Geometry check sheet. Reference: the model listing, model coordinates, mm. Face numbers are marked on the shaded views. A direction names the side the tool comes from. Give positions to 0.01 mm unless a question says otherwise; leave off trailing zeros. Order: outer loops, then holes, each group sorted by start corner. A loop starts at its lowest first (then second) coordinate and runs counter-clockwise, first axis right, second up. Notation, with made-up numbers: M 47.25,-26.5 L 61.25,-26.5 A21 cw 61.25,-13.5 Z; hole C 43,55.5 d10. An arc over 180 degrees is marked long. Answer as CSV lines item,"result".
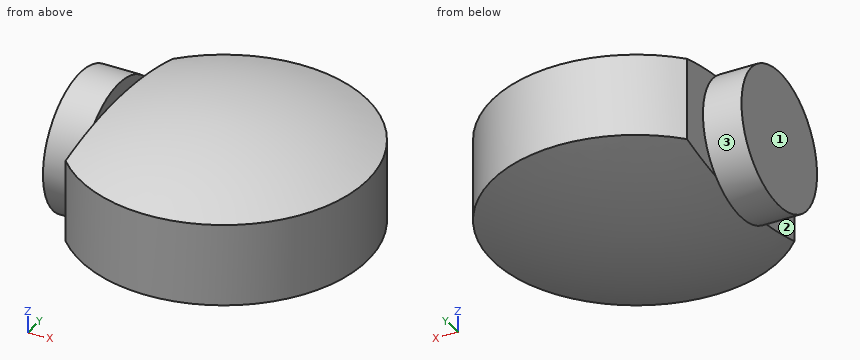
from build123d import *

# Parameters (mm, degrees)
ESQUISSE1_R           = 26
EXTRUSION1_DEPTH      = 15
D_ME1_FACE_RADIUS     = 26
D_ME1_HEIGHT          = 5
D_ME2_FACE_RADIUS     = 26
D_ME2_HEIGHT          = 5
EXTRUSION2_DEPTH      = 42.856899073
EXTRUSION2_DEPTH_BACK = 42.856899073
ESQUISSE2_W           = 16.897481419
ESQUISSE2_H           = 62.481047215
ESQUISSE3_R           = 12.5
EXTRUSION3_DEPTH      = 7


with BuildPart() as part:
    # Esquisse1 → Extrusion1 (new body)
    with BuildSketch(Plane.XY):
        Circle(ESQUISSE1_R)
    extrude(amount=EXTRUSION1_DEPTH)

    # Dôme1: a dome of height H over a round flat face of radius A is a cap of a sphere of radius (A * A + H * H) / (2 * H)
    d_me1_r = (D_ME1_FACE_RADIUS * D_ME1_FACE_RADIUS + D_ME1_HEIGHT * D_ME1_HEIGHT) / (2 * D_ME1_HEIGHT)
    d_me1_base = Plane((0, 0, 15), z_dir=(0, 0, 1))
    with Locations(d_me1_base.offset(D_ME1_HEIGHT - d_me1_r)):
        d_me1_ball = Sphere(d_me1_r, mode=Mode.PRIVATE)
    add(split(d_me1_ball, bisect_by=d_me1_base, keep=Keep.TOP, mode=Mode.PRIVATE))

    # Dôme2: a dome of height H over a round flat face of radius A is a cap of a sphere of radius (A * A + H * H) / (2 * H)
    d_me2_r = (D_ME2_FACE_RADIUS * D_ME2_FACE_RADIUS + D_ME2_HEIGHT * D_ME2_HEIGHT) / (2 * D_ME2_HEIGHT)
    d_me2_base = Plane((0, 0, 0), z_dir=(0, 0, -1))
    with Locations(d_me2_base.offset(D_ME2_HEIGHT - d_me2_r)):
        d_me2_ball = Sphere(d_me2_r, mode=Mode.PRIVATE)
    add(split(d_me2_ball, bisect_by=d_me2_base, keep=Keep.TOP, mode=Mode.PRIVATE))

    # Esquisse2 → Extrusion2 (cut, two sides: drawn at the far end of the back side and taken through both)
    with BuildSketch(Plane.XY.offset(-EXTRUSION2_DEPTH_BACK)):
        with Locations((-27.44874071, 0.855485378)):
            Rectangle(ESQUISSE2_W, ESQUISSE2_H)
    extrude(amount=EXTRUSION2_DEPTH + EXTRUSION2_DEPTH_BACK, mode=Mode.SUBTRACT)

    # Esquisse3 → Extrusion3 (add)
    with BuildSketch(Plane.ZY.offset(19)):
        with Locations(Location((7.5, -0.001760651, 0), (0, 0, 41.467990135))):
            Circle(ESQUISSE3_R)
    extrude(amount=EXTRUSION3_DEPTH)


solid = part.part
(1) Section check D-D on y = 7. Enter the section's corners in (x, z), then the cut area to 3 significant figures.
The answers:
outline,"M -26,-2.85 L -19,-2.85 L -19,-2.01 A69.75 ccw 25.04,0 L 25.04,15 A69.75 ccw -19,17.01 L -19,17.85 L -26,17.85 Z"
area,"1,110 mm2"
(2) Section check A-A on y = 1. Enter the section's corners in (x, z), then the cut area to 3 significant figures.
The answers:
outline,"M -26,-4.96 L -19,-4.96 L -19,-2.37 A70.09 ccw 25.98,0 L 25.98,15 A70.09 ccw -19,17.37 L -19,19.96 L -26,19.96 Z"
area,"1,180 mm2"
(3) Gauge pin test, flat ends, axial feed: P1, Ø3, axis at y = -9, z = -1, coming from the +X side; P2, Ø10, axis at y = 15, z = 17.5, coming from the +X side; P3, Ø12, axis at x = -6, y = 14.5, coming from the -Z side. Record the tip position at first contact, or that the pin passes through.
The answers:
P1,"stops at x = 24.78"
P2,"stops at x = 23.71"
P3,"stops at z = -4.33"
(4) Section check C-C on x = 0. Enter the section's corners in (y, z), then the cut area to 3 significant figures.
The answers:
outline,"M -26,0 A70.1 ccw 26,0 L 26,15 A70.1 ccw -26,15 Z"
area,"1,130 mm2"
(5) Section check B-B on z = 7.5. Enter the section's corners in (x, y), then the cut area to 3 significant figures.
The answers:
outline,"M -26,-12.5 L -19,-12.5 L -19,-17.75 A26 ccw long -19,17.75 L -19,12.5 L -26,12.5 Z"
area,"2,130 mm2"
(6) Material ranges on line 1 (X direction, y = -16.5, z = 7.25); line 2 (X direction, y = -19, z = 8); line 3 (Z direction, x = -17.5, y = 7), recorded low to high.
The answers:
line 1,"x = -19 to 20.09"
line 2,"x = -17.75 to 17.75"
line 3,"z = -2.42 to 17.42"
(7) Tool access check on the marked faces 1, 2 and 3. Record the directions out of +Z, -Z, +X, -X, +Y, -Y that give a thin tool (end or side, any length) a straight path to the whole face; none if there is none.
The answers:
face 1,"+Z, -Z, -X, +Y, -Y"
face 2,"-X, -Y"
face 3,"-X"
